from build123d import *

# Parameters (mm, degrees)
SKETCH024_R          = 8.5
PAD002_DEPTH         = 2.3
CHAMFER004_SIZE      = 0.75
CHAMFER005_SIZE      = 0.75
SKETCH025_R          = 9.684824
POCKET019_DEPTH      = 2.301
POCKET019_DEPTH_BACK = 0.001
SKETCH026_R          = 6
POCKET020_DEPTH      = 0.001
POCKET020_DEPTH_BACK = 2.301


with BuildPart() as part:
    # Sketch024 → Pad002 (new body)
    with BuildSketch(Plane.XY):
        Circle(SKETCH024_R)
    extrude(amount=PAD002_DEPTH)

    # Chamfer004
    chamfer004_edges = [part.edges().sort_by_distance(p)[0] for p in [
        (-8.5, 0, 2.3),
    ]]
    chamfer(chamfer004_edges, length=CHAMFER004_SIZE)

    # Chamfer005
    chamfer005_edges = [part.edges().sort_by_distance(p)[0] for p in [
        (-8.5, 0, 0),
    ]]
    chamfer(chamfer005_edges, length=CHAMFER005_SIZE)

    # Sketch025 (on Face3 of Pad002) → Pocket019 (cut, two sides)
    with BuildSketch(Plane.XY.offset(2.3)) as pocket019_sk:
        Circle(SKETCH025_R)
        Polygon((0, 8.082904), (-7, 4.041452), (-7, -4.041452), (0, -8.082904), (7, -4.041452), (7, 4.041452), align=None, mode=Mode.SUBTRACT)
    extrude(amount=-POCKET019_DEPTH, mode=Mode.SUBTRACT)
    extrude(pocket019_sk.sketch, amount=POCKET019_DEPTH_BACK, mode=Mode.SUBTRACT)

    # Sketch026 → Pocket020 (cut, two sides)
    with BuildSketch(Plane.XY) as pocket020_sk:
        Circle(SKETCH026_R)
    extrude(amount=-POCKET020_DEPTH, mode=Mode.SUBTRACT)
    extrude(pocket020_sk.sketch, amount=POCKET020_DEPTH_BACK, mode=Mode.SUBTRACT)


solid = part.part
Geometry: final body of the model. Coordinates: model frame, mm. Coordinates: 2 decimals unless noted, no trailing zeros. Order: outer loops, then holes, each group sorted by start corner. A loop starts at its lowest first (then second) coordinate and runs counter-clockwise, first axis right, second up.
1) First-contact query: P1, Ø1, axis at x = 2.5, z = 2, coming from the +Y side; P2, Ø3, axis at x = 3, y = 2, coming from the -Z side. Flat tips, straight axial feed; report the tip coordinate or a pass-through.
Result sheet:
P1: stops at y = 6.93
P2: passes through
2) Section B-B (z = 1.55). Return loops of the section in (x, y), then the cut area to 3 significant figures.
Result sheet:
outline: (-7, -4.04) - (0, -8.08) - (7, -4.04) - (7, 4.04) - (0, 8.08) - (-7, 4.04) - close; hole circle Ø12 at (0, 0)
area: 56.6 mm2
3) Section C-C (x = -1). Return loops of the section in (y, z).
Result sheet:
outline: (-7.51, 0) - (-5.92, 0) - (-5.92, 2.3) - (-7.51, 2.3) - close; (5.92, 0) - (7.51, 0) - (7.51, 2.3) - (5.92, 2.3) - close
4) Section A-A (y = 0). Return loops of the section in (x, z), then the cut area to 3 significant figures.
Result sheet:
outline: (-7, 0) - (-6, 0) - (-6, 2.3) - (-7, 2.3) - close; (6, 0) - (7, 0) - (7, 2.3) - (6, 2.3) - close
area: 4.60 mm2
5) Ray query, probe 1 along X at (y, z) = (0, 0.6); probe 2 along Y at (x, z) = (-5.5, 1.65); probe 3 along Y at (x, z) = (5, 1.7). Return the intervals inside material, ascending.
Result sheet:
probe 1: x = -7 to -6, 6 to 7
probe 2: y = -4.91 to -2.4, 2.4 to 4.91
probe 3: y = -5.2 to -3.32, 3.32 to 5.2
